CAD build for the part. Positions are in the model's coordinates, mm. A direction names the side the tool comes from. Coordinates: 2 decimals unless noted, no trailing zeros. Loops run counter-clockwise (first coordinate to the right, second up) from the corner with the lowest first, then second, coordinate; pieces in that order, holes last. Notation, with made-up numbers: (63, 48.5) -> (105, 48.5) arc R30 ccw to (105, 77.5) -> close; hole circle Ø5 at (89, -32). An arc over 180 degrees is marked (long way). Write each question's results on one line, items separated by ' | '.
```python
from build123d import *

# Parameters (mm, degrees)
F1_DEPTH = 2
F2_DEPTH = 12


with BuildPart() as f1:
    # F0 (on Top) → F1 (new body)
    with BuildSketch(Plane.XY):
        with BuildLine():
            ThreePointArc((22.608614, 24.601607), (19.679682, 31.672675), (12.608614, 34.601607))
            Line((12.608614, 34.601607), (-103.391386, 34.601607))
            ThreePointArc((-103.391386, 34.601607), (-110.462453, 31.672675), (-113.391386, 24.601607))
            Line((-113.391386, 24.601607), (-113.391386, -25.398393))
            ThreePointArc((-113.391386, -25.398393), (-110.462453, -32.469461), (-103.391386, -35.398393))
            Line((-103.391386, -35.398393), (12.608614, -35.398393))
            ThreePointArc((12.608614, -35.398393), (19.679682, -32.469461), (22.608614, -25.398393))
            Line((22.608614, -25.398393), (22.608614, 24.601607))
        make_face()
    extrude(amount=F1_DEPTH)

    # F0 (on Top) → F2 (join)
    with BuildSketch(Plane.XY):
        with BuildLine():
            ThreePointArc((26.608614, 28.601607), (23.679682, 35.672675), (16.608614, 38.601607))
            Line((16.608614, 38.601607), (-107.391386, 38.601607))
            ThreePointArc((-107.391386, 38.601607), (-114.462453, 35.672675), (-117.391386, 28.601607))
            Line((-117.391386, 28.601607), (-117.391386, -29.398393))
            ThreePointArc((-117.391386, -29.398393), (-114.462453, -36.469461), (-107.391386, -39.398393))
            Line((-107.391386, -39.398393), (16.608614, -39.398393))
            ThreePointArc((16.608614, -39.398393), (23.679682, -36.469461), (26.608614, -29.398393))
            Line((26.608614, -29.398393), (26.608614, 28.601607))
        make_face()
        with BuildLine():
            Line((-103.391386, 34.601607), (12.608614, 34.601607))
            ThreePointArc((12.608614, 34.601607), (19.679682, 31.672675), (22.608614, 24.601607))
            Line((22.608614, 24.601607), (22.608614, -25.398393))
            ThreePointArc((22.608614, -25.398393), (19.679682, -32.469461), (12.608614, -35.398393))
            Line((12.608614, -35.398393), (-103.391386, -35.398393))
            ThreePointArc((-103.391386, -35.398393), (-110.462453, -32.469461), (-113.391386, -25.398393))
            Line((-113.391386, -25.398393), (-113.391386, 24.601607))
            ThreePointArc((-113.391386, 24.601607), (-110.462453, 31.672675), (-103.391386, 34.601607))
        make_face(mode=Mode.SUBTRACT)
    extrude(amount=F2_DEPTH)


solid = f1.part
```
Q1. Which spindle directions (+Z, -Z, +X, -X, +Y, -Y) get a long thin tool onto all of the face, cutting with end or side? Do faces 4 (the flat face through (-46, 0, 0)), 5 (the flat face through (-46, 0, 2)). Say none if no direction does.
Results are:
face 4: -Z, +X, -X, +Y, -Y | face 5: +Z
Q2. Wall check: L1, parallel to X at y = -10.5, z = 8.5; L2, parallel to Y at x = -57.5, z = 6; L3, parallel to Z at x = -68.5, y = 14. Give the ranges that are in metal, low to high. Write a range as from..to.
Results are:
L1: -117.39..-113.39, 22.61..26.61 | L2: -39.4..-35.4, 34.6..38.6 | L3: 0..2
Q3. Pull direction Y, two halves, no side cores. Call faces 1 (the cylindrical face through (-114.384, 35.75, 5.916)), 2 (the flat face through (-46, -39.398, 6)), 3 (the cylindrical face through (-110.54, 31.594, 6.93)): +Y half, -Y half, draft (parallel to the pull), parting line (faces both ways), or undercut.
Results are:
face 1: +Y half | face 2: -Y half | face 3: undercut
Q4. Drop a flat-ended pin along its axis: pin 1 (3 mm diameter, centred on x = -60, y = 2, fed in from +Z). Give the stop position or say it passes through.
Results are:
pin 1: z = 2
Q5. Cut at A-A on z = 3.5. Write the cut outline in (x, y), and give its area (3 significant figures).
Results are:
outline: (-117.39, -29.4) arc R10 ccw to (-107.39, -39.4) -> (16.61, -39.4) arc R10 ccw to (26.61, -29.4) -> (26.61, 28.6) arc R10 ccw to (16.61, 38.6) -> (-107.39, 38.6) arc R10 ccw to (-117.39, 28.6) -> close; hole (-113.39, -25.4) arc R10 ccw to (-103.39, -35.4) -> (12.61, -35.4) arc R10 ccw to (22.61, -25.4) -> (22.61, 24.6) arc R10 ccw to (12.61, 34.6) -> (-103.39, 34.6) arc R10 ccw to (-113.39, 24.6) -> close | area: 1,710 mm^2
Q6. Cut at B-B on x = -87. Write the cut outline in (y, z), and give its area (3 significant figures).
Results are:
outline: (-39.4, 0) -> (38.6, 0) -> (38.6, 12) -> (34.6, 12) -> (34.6, 2) -> (-35.4, 2) -> (-35.4, 12) -> (-39.4, 12) -> close | area: 236 mm^2
Q7. Cut at C-C on y = 16. Write the cut outline in (x, z).
Results are:
outline: (-117.39, 0) -> (26.61, 0) -> (26.61, 12) -> (22.61, 12) -> (22.61, 2) -> (-113.39, 2) -> (-113.39, 12) -> (-117.39, 12) -> close
